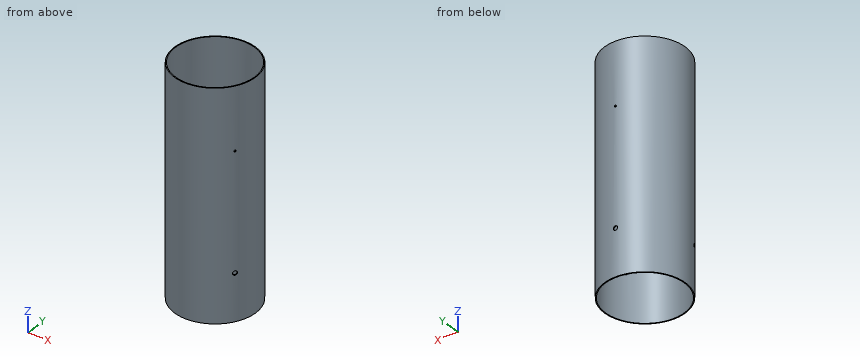
```python
from build123d import *

# Parameters (mm, degrees)
SKETCH1_R                = 49.6697
SKETCH1_R_2              = 48.5394
BOSS_EXTRUDE1_DEPTH      = 276.225
SKETCH2_R                = 2.6289
SKETCH2_R_2              = 1.143
F_8_32_T_NUT_HOLES_DEPTH = 5.08
CIRPATTERN1_COUNT        = 3


with BuildPart() as part:
    # Sketch1 → Boss-Extrude1 (new body)
    with BuildSketch(Plane.XY):
        Circle(SKETCH1_R)
        Circle(SKETCH1_R_2, mode=Mode.SUBTRACT)
    extrude(amount=BOSS_EXTRUDE1_DEPTH)

    # Sketch2 → 8-32 T-Nut Holes (cut)
    with BuildSketch(Plane(origin=(0, 49.6697, 0), x_dir=(1, 0, 0), z_dir=(0, 1, 0))):
        with Locations(Location((0, -57.15, 0), (0, 0, 270))):
            Circle(SKETCH2_R)
        with Locations(Location((0, -200.025, 0), (0, 0, 270))):
            Circle(SKETCH2_R_2)
    f_8_32_t_nut_holes = extrude(amount=-F_8_32_T_NUT_HOLES_DEPTH, mode=Mode.SUBTRACT)

    # CirPattern1: 8-32 T-Nut Holes ×3 about axis
    cirpattern1_axis = Axis((0, 0, 276.225), (0, 0, -1))
    for i in range(1, CIRPATTERN1_COUNT):
        add(f_8_32_t_nut_holes.rotate(cirpattern1_axis, i * 360 / CIRPATTERN1_COUNT), mode=Mode.SUBTRACT)


solid = part.part
```
Source: CAD feature listing. Evaluate the final solid. Frame: model axes, mm. Coordinates: 2 decimals unless noted, no trailing zeros. Order: outer loops, then holes, each group sorted by start corner. A loop starts at its lowest first (then second) coordinate and runs counter-clockwise, first axis right, second up. Notation, with made-up numbers: (-18.75, -10.75) - (36.25, -10.75) arc R15 ccw to (36.25, 7.25) - close; hole circle Ø6 at (60, 73.25). An arc over 180 degrees is marked (long way). One line per item, written item: value.
1) Cut plane A-A on y = 0. Output: boundary loops of the cut face in (x, z) (3 decimals), plus the area to 3 significant figures.
Computed values:
outline: (-49.67, 0) - (-48.539, 0) - (-48.539, 276.225) - (-49.67, 276.225) - close; (48.539, 0) - (49.67, 0) - (49.67, 276.225) - (48.539, 276.225) - close
area: 624 mm^2
2) Contact query for flat-ended pins moving along their axis: pin 1 (2.5 mm diameter, centred on x = 0, z = 200.025, fed in from -Y); pin 2 (10 mm diameter, centred on y = 16, z = 79.5, fed in from -X); pin 3 (3 mm diameter, centred on x = 0, z = 57.15, fed in from +Y). Output: stop coordinate, or through.
Computed values:
pin 1: stops at y = -49.67
pin 2: stops at x = -48.44
pin 3: stops at y = -48.52
3) Ray query, line 1 (Z direction, x = 0, y = 48.8) (3 decimals); line 2 (Y direction, x = 1, z = 45); line 3 (Y direction, x = -10.5, z = 227). Return the intervals inside material, ascending. Write a range as [from, to].
Computed values:
line 1: z = [0, 54.521], [59.779, 198.882], [201.168, 276.225]
line 2: y = [-49.66, -48.53], [48.53, 49.66]
line 3: y = [-48.55, -47.39], [47.39, 48.55]
4) Cut plane C-C on x = -10. Output: boundary loops of the cut face in (y, z) (3 decimals).
Computed values:
outline: (-48.653, 0) - (-47.498, 0) - (-47.498, 276.225) - (-48.653, 276.225) - close; (47.498, 0) - (48.653, 0) - (48.653, 276.225) - (47.498, 276.225) - close
5) Cut plane B-B on z = 57.15. Output: boundary loops of the cut face in (x, y), plus the area to 3 significant figures.
Computed values:
outline: (-44.27, -22.52) - (-43.29, -21.96) arc R48.54 cw to (-2.63, 48.47) - (-2.63, 49.6) arc R49.67 ccw to start; (-41.64, -27.08) arc R49.67 ccw to (41.64, -27.08) - (40.66, -26.51) arc R48.54 cw to (-40.66, -26.51) - close; (2.63, 48.47) arc R48.54 cw to (43.29, -21.96) - (44.27, -22.52) arc R49.67 ccw to (2.63, 49.6) - close
area: 331 mm^2
